```python
from build123d import *

# Parameters (mm, degrees)
SKETCH_1_R               = 11.35
EXTRUDE_1_DEPTH          = 8
SKETCH_2_R               = 13.95
EXTRUDE_2_DEPTH          = 2
EXTRUDE_START            = 2
SKETCH_3_R               = 13.95
EXTRUDE_3_DEPTH          = 2
SKETCH_4_R               = 2.5
CUT_EXTRUDE_1_DEPTH      = 29.09279267
SKETCH_5_R               = 2
CUT_EXTRUDE_2_DEPTH      = 23.117979112
SKETCH_6_W               = 2.4
SKETCH_6_H               = 16
CUT_EXTRUDE_3_DEPTH      = 1.2
PATTERN_CIRCULAR_1_COUNT = 15


with BuildPart() as part:
    # 草图1 → 凸台-拉伸1 (new, symmetric)
    with BuildSketch(Plane(origin=(0, 0, 0), x_dir=(1, 0, 0), z_dir=(0, 1, 0))):
        with Locations(Location((0, 0, 0), (0, 0, 270))):
            Circle(SKETCH_1_R)
    extrude(amount=EXTRUDE_1_DEPTH, both=True)

    # 草图2 → 凸台-拉伸2 (add)
    with BuildSketch(Plane(origin=(0, 8, 0), x_dir=(1, 0, 0), z_dir=(0, 1, 0))):
        with Locations(Location((0, 0, 0), (0, 0, 270))):
            Circle(SKETCH_2_R)
    extrude(amount=EXTRUDE_2_DEPTH)

    # 草图3 → 凸台-拉伸3 (add)
    with BuildSketch(Plane.XZ.offset(8).offset(EXTRUDE_START)):
        with Locations(Location((0, 0, 0), (0, 0, 90))):
            Circle(SKETCH_3_R)
    extrude(amount=-EXTRUDE_3_DEPTH)

    # 草图4 → 切除-拉伸1 (cut, through all)
    with BuildSketch(Plane(origin=(0, 10, 0), x_dir=(1, 0, 0), z_dir=(0, 1, 0))):
        with Locations(Location((0, 0, 0), (0, 0, 270))):
            Circle(SKETCH_4_R)
    extrude(amount=-CUT_EXTRUDE_1_DEPTH, mode=Mode.SUBTRACT)

    # 草图5 → 切除-拉伸2 (cut, through all)
    with BuildSketch(Plane.XY):
        with Locations(Location((0, 0, 0), (0, 0, 90.000000031))):
            Circle(SKETCH_5_R)
    extrude(amount=CUT_EXTRUDE_2_DEPTH, mode=Mode.SUBTRACT)

    # 草图6 → 切除-拉伸3 (cut, symmetric)
    with BuildSketch(Plane.XY):
        with Locations((11.35, 0)):
            Rectangle(SKETCH_6_W, SKETCH_6_H)
    cut_extrude_3 = extrude(amount=CUT_EXTRUDE_3_DEPTH, both=True, mode=Mode.SUBTRACT)

    # 阵列(圆周)1: 切除-拉伸3 ×15 about axis
    pattern_circular_1_axis = Axis((0, 0, 0), (0, 1, 0))
    for i in range(1, PATTERN_CIRCULAR_1_COUNT):
        add(cut_extrude_3.rotate(pattern_circular_1_axis, i * 360 / PATTERN_CIRCULAR_1_COUNT), mode=Mode.SUBTRACT)


solid = part.part
```
Verification items for the finished model (mm, model axes). A direction names the side the tool comes from. Round coordinates to 2 decimals unless told otherwise and drop trailing zeros. Write each loop counter-clockwise with the first axis right and the second up, starting at its lowest first coordinate (ties: lowest second). Pieces come first, ordered by that corner, then holes. Notation, with made-up numbers: (-23, 12) -> (-18, 12) arc R17 ccw to (-18, 34) -> close; hole circle Ø7 at (-37.75, 64). An arc over 180 degrees is marked (long way). Write each question's results on one line, items separated by ' | '. Start each with the question number.
1. Draft check along Z on faces 5 (the flat face through (8.1, 0.1, 7.2)), 6 (the flat face through (0.074, 0.112, -10.777)), 7 (the cylindrical face through (1.203, 0.112, -11.286)). Enter one of: +Z half, -Z half, draft (parallel to the pull), parting line (faces both ways), or undercut.
2. Cross-section at A-A (z = 0). Enter the section's corners in (x, y), then the cut area to 3 significant figures.
3. Cross-section at B-B (x = 3.5). Enter the section's corners in (y, z), then the cut area to 3 significant figures.
4. Depth check by flat-ended pin: P1, Ø4, axis at y = 2, z = 1, coming from the +X side; P2, Ø1, axis at x = -9, y = -4.5, coming from the -Z side; P3, Ø1.2, axis at y = 0, z = -0.5, coming from the +X side; P4, Ø2, axis at x = -1, z = -2, coming from the -Y side. Enter the tip coordinate at first touch or a pass-through.
5. Material ranges on probe 1 along Y at (x, z) = (6.25, 10.5); probe 2 along X at (y, z) = (0, 5.5); probe 3 along Y at (x, z) = (1.5, 3.75), recorded low to high. Write a range as from..to.
6. Set-up check for faces 1 (the flat face through (-2.313, 0.112, -10.526)), 2 (the flat face through (11, 0, 1.2)), 3 (the cylindrical face through (-7.58, 0.11, -8.45)), 4 (the flat face through (-2.313, 0.112, 10.526)): record each of +Z, -Z, +X, -X, +Y, -Y from which the full face is reachable in a straight line by a thin tool's end or side.
7. Cross-section at C-C (z = 12.25). Enter the section's corners in (x, y).
Solutions:
1) face 5: +Z half | face 6: undercut | face 7: -Z half
2) outline: (-13.95, -10) -> (-2.5, -10) -> (-2.5, 10) -> (-13.95, 10) -> (-13.95, 8) -> (-11.35, 8) -> (-11.35, -8) -> (-13.95, -8) -> close; (2.5, -10) -> (13.95, -10) -> (13.95, -8) -> (10.15, -8) -> (10.15, 8) -> (13.95, 8) -> (13.95, 10) -> (2.5, 10) -> close | area: 356 mm2
3) outline: (-10, -13.5) -> (-8, -13.5) -> (-8, -9.54) -> (8, -9.54) -> (8, -13.5) -> (10, -13.5) -> (10, 13.5) -> (8, 13.5) -> (8, 9.54) -> (-8, 9.54) -> (-8, 13.5) -> (-10, 13.5) -> close | area: 413 mm2
4) P1: stops at x = 11.29 | P2: stops at z = -5.57 | P3: stops at x = 10.15 | P4: stops at y = -10
5) probe 1: y = -10..-8, 8..10 | probe 2: x = -9.93..-9.61, -8.55..-2, 2..9.4 | probe 3: y = -10..-1.32, 1.32..10
6) face 1: -Z | face 2: +X | face 3: -Z, -X | face 4: +Z
7) outline: (-6.67, -10) -> (6.67, -10) -> (6.67, -8) -> (-6.67, -8) -> close; (-6.67, 8) -> (6.67, 8) -> (6.67, 10) -> (-6.67, 10) -> close
